Autodesk Inventor part; units mm, degrees
ref_plane "YZ Plane" through (0, 0, 0) normal (1, 0, 0) x (0, 1, 0)
ref_plane "XZ Plane" through (0, 0, 0) normal (0, 1, 0) x (-1, 0, 0)
ref_plane "XY Plane" through (0, 0, 0) normal (0, 0, 1) x (1, 0, 0)
sketch "Sketch1" plane through (0, 0, 0) normal (0, 1, 0) x (-1, 0, 0)
  line L0 (0, 0) -> (-90.17, 0)
  line L1 (-90.17, 0) -> (-90.17, -66.04)
  line L2 (-90.17, -66.04) -> (0, -66.04)
  line L3 (0, -66.04) -> (0, 0)
  dimension "d0" = 90.17
  dimension "d1" = 66.04
extrude "Extrusion1" add sketch "Sketch1" along normal blind 5.08
sketch "Sketch2" plane through (0, 0, 0) normal (0, -1, 0) x (1, 0, 0)
  circle A0 centre (8.9218, -8.9217) radius 5.8738
  circle A1 centre (81.2483, -8.9218) radius 5.8738
  circle A2 centre (8.9217, -57.1183) radius 5.8738
  circle A3 centre (81.2483, -57.1183) radius 5.8738
  line L0 (0, 0) -> (90.17, 0)
  line L1 (0, -66.04) -> (0, 0)
  line L2 (90.17, -66.04) -> (0, -66.04)
  line L3 (90.17, 0) -> (90.17, -66.04)
  dimension "d4" = 11.7475
  dimension "d5" = 3.048
  dimension "d6" = 3.048
  dimension "d7" = 3.048
  dimension "d8" = 3.048
extrude "Extrusion2" add sketch "Sketch2" along normal blind 2.5908 contours A0 | A1 | A2 | A3
sketch "Sketch3" plane through (0, 0, 0) normal (0, -1, 0) x (1, 0, 0)
  line L0 (78.6638, -30.099) -> (78.6638, -35.941) construction
  line L1 (73.5838, -30.099) -> (73.5838, -35.941)
  line L2 (83.7438, -35.941) -> (83.7438, -30.099)
  arc A0 (83.7438, -30.099) -> (73.5838, -30.099) centre (78.6638, -30.099) ccw
  arc A1 (73.5838, -35.941) -> (83.7438, -35.941) centre (78.6638, -35.941) ccw
  line L3 (11.5062, -30.099) -> (11.5062, -35.941) construction
  line L4 (6.4262, -30.099) -> (6.4262, -35.941)
  line L5 (16.5862, -35.941) -> (16.5862, -30.099)
  arc A2 (16.5862, -30.099) -> (6.4262, -30.099) centre (11.5062, -30.099) ccw
  arc A3 (6.4262, -35.941) -> (16.5862, -35.941) centre (11.5062, -35.941) ccw
  line L6 (90.17, 0) -> (90.17, -66.04)
  line L7 (0, -66.04) -> (0, 0)
  point P0 (78.6638, -33.02)
  point P1 (11.5062, -33.02)
  point P2 (90.17, -33.02)
  dimension "d11" = 6.4262
  dimension "d12" = 10.16
  dimension "d14" = 6.4262
  dimension "d15" = 16.002
extrude "Extrusion3" add sketch "Sketch3" along normal blind 4.064
sketch "Sketch4" plane through (0, -4.064, 0) normal (0, -1, 0) x (1, 0, 0)
  point P0 (0, 0)
sketch "Sketch5" plane through (0, -4.064, 0) normal (0, -1, 0) x (1, 0, 0)
  circle A0 centre (78.6638, -35.941) radius 4.1275
  circle A1 centre (11.5062, -35.941) radius 4.1275
  arc A2 (6.4262, -35.941) -> (16.5862, -35.941) centre (11.5062, -35.941) ccw
  arc A3 (73.5838, -35.941) -> (83.7438, -35.941) centre (78.6638, -35.941) ccw
  line L0 (11.5062, -35.941) -> (11.5062, -30.099) construction
  line L1 (14.4272, -35.941) -> (14.4272, -30.099)
  line L2 (8.5852, -30.099) -> (8.5852, -35.941)
  arc A4 (8.5852, -35.941) -> (14.4272, -35.941) centre (11.5062, -35.941) ccw
  arc A5 (14.4272, -30.099) -> (8.5852, -30.099) centre (11.5062, -30.099) ccw
  line L3 (78.6638, -35.941) -> (78.6638, -30.099) construction
  line L4 (81.5848, -35.941) -> (81.5848, -30.099)
  line L5 (75.7428, -30.099) -> (75.7428, -35.941)
  arc A6 (75.7428, -35.941) -> (81.5848, -35.941) centre (78.6638, -35.941) ccw
  arc A7 (81.5848, -30.099) -> (75.7428, -30.099) centre (78.6638, -30.099) ccw
  arc A8 (16.5862, -30.099) -> (6.4262, -30.099) centre (11.5062, -30.099) ccw
  point P0 (0, 0)
  point P1 (11.5062, -33.02)
  point P2 (78.6638, -33.02)
  dimension "d18" = 5.842
  dimension "d19" = 8.255
extrude "Extrusion4" cut sketch "Sketch5" against normal blind 8.89
fillet "Fillet1" radius 12.7 4 edges at (90.17, 2.54, 0) (90.17, 2.54, -66.04) (0, 2.54, 0) (0, 2.54, -66.04)
sketch "Sketch6" plane through (0, 4.826, 0) normal (0, -1, 0) x (1, 0, 0)
  circle A0 centre (11.5062, -30.099) radius 2.286
  arc A1 (14.4272, -30.099) -> (8.5852, -30.099) centre (11.5062, -30.099) ccw
  circle A2 centre (78.6638, -30.099) radius 2.286
  arc A3 (81.5848, -30.099) -> (75.7428, -30.099) centre (78.6638, -30.099) ccw
  point P0 (0, 0)
  dimension "d23" = 4.572
  dimension "d24" = 4.572
extrude "Extrusion5" add sketch "Sketch6" along normal blind 19.05
equation "\"d6\" = d5"
equation "\"d7\" = d5"
equation "\"d8\" = d5"
equation "\"d14\" = d11"
properties part number "Router Bottom"
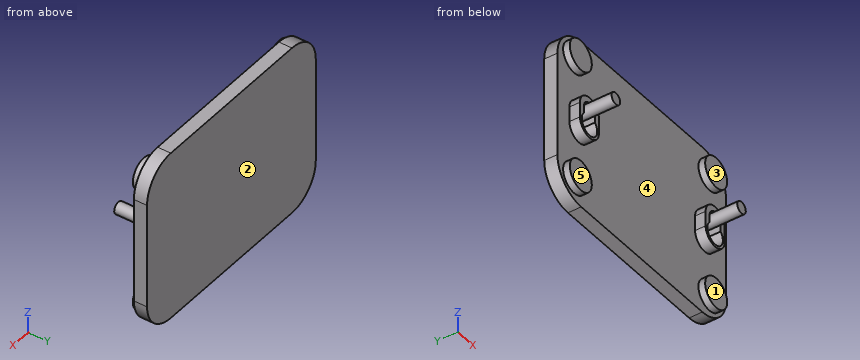
CAD build for the part. Positions are in the model's coordinates, mm. Face numbers are marked on the shaded views. A direction names the side the tool comes from. Give positions to 0.01 mm unless a question says otherwise; leave off trailing zeros. Loops run counter-clockwise (first coordinate to the right, second up) from the corner with the lowest first, then second, coordinate; pieces in that order, holes last. Notation, with made-up numbers: M 49.5,69.5 L 82.5,69.5 A23 cw 82.5,100.5 Z; hole C 20.5,8.25 d2. An arc over 180 degrees is marked long. Use one line per item in the form item = value.
Item 1: Flat gauge pins, fed straight in: pin 1 (1.2 mm diameter, centred on y = -2, z = -33.5, fed in from -X); pin 2 (1.5 mm diameter, centred on x = 36, z = -40, fed in from -Y); pin 3 (1.2 mm diameter, centred on y = -1.5, z = -33.5, fed in from +X). Where does each tip first touch, or does it go through?
Determined:
pin_1 = 6.43
pin_2 = 0
pin_3 = 83.74
Item 2: Slice it at A-A (y = -10). List the corners of the cut face in (x, z).
Determined:
outline = C 11.51,-30.1 d4.57; C 78.66,-30.1 d4.57
Item 3: Slice it at D-D (z = -56). List the corners of the cut face in (x, y), plus the area to 3 significant figures.
Determined:
outline = M 0.28,0 L 3.16,0 L 3.16,-2.59 L 14.69,-2.59 L 14.69,0 L 75.48,0 L 75.48,-2.59 L 87.01,-2.59 L 87.01,0 L 89.89,0 L 89.89,5.08 L 0.28,5.08 Z
area = 515 mm2
Item 4: Slice it at C-C (x = 25). List the corners of the cut face in (y, z), plus the area to 3 significant figures.
Determined:
outline = M 0,-66.04 L 5.08,-66.04 L 5.08,0 L 0,0 Z
area = 335 mm2
Item 5: Which spindle directions (+Z, -Z, +X, -X, +Y, -Y) get a long thin tool onto all of the face, cutting with end or side? Do the marked faces 1, 2 and 3. Say none if no direction does.
Determined:
face_1 = -Z, +X, -X, -Y
face_2 = +Z, -Z, +X, -X, +Y
face_3 = +Z, +X, -X, -Y
Item 6: Drill centre lines: probe 1 along Y at (x, z) = (30.5, -20); probe 2 along X at (y, z) = (-9.5, -30); probe 3 along Y at (x, z) = (82.5, -32.5). Where is each one in solid material? Low to high. Write a range as from..to.
Determined:
probe_1 = 0..5.08
probe_2 = 9.22..13.79, 76.38..80.95
probe_3 = -4.06..5.08
Item 7: Slice it at B-B (z = -37). List the corners of the cut face in (x, y), plus the area to 3 significant figures.
Determined:
outline = M 0,0 L 6.54,0 L 6.54,-4.06 L 7.52,-4.06 L 7.52,4.83 L 15.5,4.83 L 15.5,-4.06 L 16.47,-4.06 L 16.47,0 L 73.7,0 L 73.7,-4.06 L 74.67,-4.06 L 74.67,4.83 L 82.65,4.83 L 82.65,-4.06 L 83.63,-4.06 L 83.63,0 L 90.17,0 L 90.17,5.08 L 0,5.08 Z
area = 397 mm2
Item 8: Two-plate mould, pull along Z, no slides. Class the marked faces 4 and 5: pulls with the +Z half, pulls with the -Z half, needs draft (parallel to the pull), parting line crosses it, or undercut.
Determined:
face_4 = undercut
face_5 = needs draft
